Can you work these out from the model? Positions are in its coordinate system, mm. Face numbers are marked on the shaded views. A direction names the side the tool comes from. Coordinates: 2 decimals unless noted, no trailing zeros. Order: outer loops, then holes, each group sorted by start corner. A loop starts at its lowest first (then second) coordinate and runs counter-clockwise, first axis right, second up. Notation, with made-up numbers: (47, 44) -> (96, 44) arc R29 cw to (96, 80) -> close; hole circle Ø3 at (72, 48). An arc over 180 degrees is marked (long way). Use a Markdown table: item, result. Add a question column.
1. Suppose I cut it at C-C, the plane y = 9. State how many separate pieces and enclosed holes the cut face has, then the cut area to 3 significant figures.
2. Suppose I cut it at A-A, the plane z = 11. List the corners of the cut face in (x, y) for me, then the cut area to 3 significant figures.
3. For the marked faces 3, 4 and 5, which set-ups out of +Z, -Z, +X, -X, +Y, -Y let a thin tool reach every point of the face, with its end or its side?
4. Suppose I cut it at D-D, the plane z = -26.5. List the corners of the cut face in (x, y) for me.
5. If I drill on line 1 along Z through (x, y) = (87, 9.75); line 2 along Y through (x, z) = (11, -15.5); line 3 along Y through (x, z) = (52, -1), over which ranges is the centre line in solid material (lowest first)? Write a range as from..to.
6. We'd pull the mould along X, two halves only. Please class the marked faces 1 and 2: pulls with the +X half, pulls with the -X half, needs draft (parallel to the pull), parting line crosses it, or undercut.
7. Suppose I cut it at B-B, the plane x = 64.5. List the corners of the cut face in (y, z) for me.
8. For pin 1 Ø5 at (x, z) = (52, 6.5) entering from +Y; pin 2 Ø0.9 at (x, y) = (67.5, 7) entering from -Z; pin 3 Ø2 at (x, y) = (55, 3) entering from -Z; pin 4 Ø3 at (x, y) = (47.5, 2) entering from +Z, each with a flat end and sliding along its axis, tell me the tip position at first contact or that it passes through.
```python
from build123d import *

# Parameters (mm, degrees)
SKETCH1_W            = 100
SKETCH1_H            = 16
BOSS_EXTRUDE1_DEPTH  = 3
SKETCH2_W            = 98
SKETCH2_H            = 14
CUT_EXTRUDE1_DEPTH   = 1
SKETCH5_W            = 20
SKETCH5_H            = 3
BOSS_EXTRUDE4_DEPTH  = 15
SKETCH6_W            = 20
SKETCH6_H            = 3
BOSS_EXTRUDE5_DEPTH  = 15
FILLET18_R           = 10
SKETCH7_W            = 3
SKETCH7_H            = 12
BOSS_EXTRUDE6_DEPTH  = 17
SKETCH8_W            = 6
SKETCH8_H            = 2
BOSS_EXTRUDE7_DEPTH  = 2
FILLET19_R           = 6
SKETCH10_W           = 60
SKETCH10_H           = 3
BOSS_EXTRUDE8_DEPTH  = 3
SKETCH11_W           = 60
SKETCH11_H           = 3
BOSS_EXTRUDE9_DEPTH  = 3
SKETCH12_W           = 0.95
SKETCH12_H           = 14
BOSS_EXTRUDE10_DEPTH = 3
SKETCH13_W           = 100
SKETCH13_H           = 0.95
BOSS_EXTRUDE11_DEPTH = 3
SKETCH14_W           = 0.95
SKETCH14_H           = 0.052088128
BOSS_EXTRUDE12_DEPTH = 3
SKETCH15_W           = 0.95
SKETCH15_H           = 0.047911872
SKETCH15_W_2         = 0.949734752
SKETCH15_H_2         = 0.052088128
BOSS_EXTRUDE13_DEPTH = 3
FILLET20_R           = 10
SKETCH17_W           = 98.1
SKETCH17_H           = 14.1
SKETCH17_W_2         = 97.1
SKETCH17_H_2         = 13.1
CUT_EXTRUDE2_DEPTH   = 4
SKETCH18_W           = 100
SKETCH18_H           = 16.05
SKETCH18_W_2         = 98
SKETCH18_H_2         = 14.05
CUT_EXTRUDE3_DEPTH   = 2
SKETCH19_W           = 100
SKETCH19_H           = 16
SKETCH19_W_2         = 98.1
SKETCH19_H_2         = 14.1
BOSS_EXTRUDE14_DEPTH = 1


with BuildPart() as part:
    # Sketch1 → Boss-Extrude1 (new body)
    with BuildSketch(Plane(origin=(0, 0, 0), x_dir=(1, 0, 0), z_dir=(0, 1, 0))):
        with Locations((50, 8)):
            Rectangle(SKETCH1_W, SKETCH1_H)
    extrude(amount=BOSS_EXTRUDE1_DEPTH)

    # Sketch2 → Cut-Extrude1 (cut)
    with BuildSketch(Plane(origin=(0, 3, 0), x_dir=(1, 0, 0), z_dir=(0, 1, 0))):
        with Locations((50, 8)):
            Rectangle(SKETCH2_W, SKETCH2_H)
    extrude(amount=-CUT_EXTRUDE1_DEPTH, mode=Mode.SUBTRACT)

    # Sketch5 → Boss-Extrude4 (add)
    with BuildSketch(Plane.XY):
        with Locations((10, 1.5)):
            Rectangle(SKETCH5_W, SKETCH5_H)
        with Locations((90, 1.5)):
            Rectangle(SKETCH5_W, SKETCH5_H)
    extrude(amount=BOSS_EXTRUDE4_DEPTH)

    # Sketch6 → Boss-Extrude5 (add)
    with BuildSketch(Plane(origin=(0, 0, -16), x_dir=(-1, 0, 0), z_dir=(0, 0, -1))):
        with Locations((-90, 1.5)):
            Rectangle(SKETCH6_W, SKETCH6_H)
        with Locations((-10, 1.5)):
            Rectangle(SKETCH6_W, SKETCH6_H)
    extrude(amount=BOSS_EXTRUDE5_DEPTH)

    # Fillet18
    fillet18_edges = [part.edges().sort_by_distance(p)[0] for p in [
        (20, 1.5, 15),
        (0, 1.5, 15),
        (80, 1.5, 15),
        (100, 1.5, 15),
        (0, 1.5, -31),
        (20, 1.5, -31),
        (80, 1.5, -31),
        (100, 1.5, -31),
    ]]
    fillet(fillet18_edges, radius=FILLET18_R - 0.0001)  # a hair under: the kernel refuses the full size

    # Sketch7 → Boss-Extrude6 (add)
    with BuildSketch(Plane(origin=(0, 2, 0), x_dir=(1, 0, 0), z_dir=(0, 1, 0))):
        with Locations((95, 8)):
            Rectangle(SKETCH7_W, SKETCH7_H)
        with Locations((86, 8)):
            Rectangle(SKETCH7_W, SKETCH7_H)
        with Locations((77, 8)):
            Rectangle(SKETCH7_W, SKETCH7_H)
        with Locations((68, 8)):
            Rectangle(SKETCH7_W, SKETCH7_H)
        with Locations((59, 8)):
            Rectangle(SKETCH7_W, SKETCH7_H)
        with Locations((50, 8)):
            Rectangle(SKETCH7_W, SKETCH7_H)
        with Locations((41, 8)):
            Rectangle(SKETCH7_W, SKETCH7_H)
        with Locations((32, 8)):
            Rectangle(SKETCH7_W, SKETCH7_H)
        with Locations((23, 8)):
            Rectangle(SKETCH7_W, SKETCH7_H)
        with Locations((14, 8)):
            Rectangle(SKETCH7_W, SKETCH7_H)
        with Locations((5, 8)):
            Rectangle(SKETCH7_W, SKETCH7_H)
    extrude(amount=BOSS_EXTRUDE6_DEPTH)

    # Sketch8 → Boss-Extrude7 (add)
    with BuildSketch(Plane(origin=(0, 2, 0), x_dir=(1, 0, 0), z_dir=(0, 1, 0))):
        with Locations((90.5, 8)):
            Rectangle(SKETCH8_W, SKETCH8_H)
        with Locations((81.5, 8)):
            Rectangle(SKETCH8_W, SKETCH8_H)
        with Locations((72.5, 8)):
            Rectangle(SKETCH8_W, SKETCH8_H)
        with Locations((63.5, 8)):
            Rectangle(SKETCH8_W, SKETCH8_H)
        with Locations((54.5, 8)):
            Rectangle(SKETCH8_W, SKETCH8_H)
        with Locations((45.5, 8)):
            Rectangle(SKETCH8_W, SKETCH8_H)
        with Locations((36.5, 8)):
            Rectangle(SKETCH8_W, SKETCH8_H)
        with Locations((27.5, 8)):
            Rectangle(SKETCH8_W, SKETCH8_H)
        with Locations((18.5, 8)):
            Rectangle(SKETCH8_W, SKETCH8_H)
        with Locations((9.5, 8)):
            Rectangle(SKETCH8_W, SKETCH8_H)
    extrude(amount=BOSS_EXTRUDE7_DEPTH)

    # Fillet19
    fillet19_edges = [part.edges().sort_by_distance(p)[0] for p in [
        (95, 19, -2),
        (95, 19, -14),
        (86, 19, -2),
        (86, 19, -14),
        (77, 19, -2),
        (77, 19, -14),
        (68, 19, -2),
        (68, 19, -14),
        (59, 19, -2),
        (59, 19, -14),
        (50, 19, -2),
        (50, 19, -14),
        (41, 19, -2),
        (41, 19, -14),
        (32, 19, -2),
        (32, 19, -14),
        (23, 19, -14),
        (23, 19, -2),
        (14, 19, -2),
        (14, 19, -14),
        (5, 19, -2),
        (5, 19, -14),
    ]]
    fillet(fillet19_edges, radius=FILLET19_R - 0.0001)  # a hair under: the kernel refuses the full size

    # Sketch10 → Boss-Extrude8 (add)
    with BuildSketch(Plane(origin=(0, 0, -16), x_dir=(-1, 0, 0), z_dir=(0, 0, -1))):
        with Locations((-50, 1.5)):
            Rectangle(SKETCH10_W, SKETCH10_H)
    extrude(amount=BOSS_EXTRUDE8_DEPTH)

    # Sketch11 → Boss-Extrude9 (add)
    with BuildSketch(Plane.XY):
        with Locations((50, 1.5)):
            Rectangle(SKETCH11_W, SKETCH11_H)
    extrude(amount=BOSS_EXTRUDE9_DEPTH)

    # Sketch12 → Boss-Extrude10 (add)
    with BuildSketch(Plane(origin=(0, 3, 0), x_dir=(1, 0, 0), z_dir=(0, 1, 0))):
        with Locations((99.525, 7.997911872)):
            Rectangle(SKETCH12_W, SKETCH12_H)
        with Locations((0.475, 7.997911872)):
            Rectangle(SKETCH12_W, SKETCH12_H)
    extrude(amount=BOSS_EXTRUDE10_DEPTH)

    # Sketch13 → Boss-Extrude11 (add)
    with BuildSketch(Plane(origin=(0, 3, 0), x_dir=(1, 0, 0), z_dir=(0, 1, 0))):
        with Locations((50, 15.525)):
            Rectangle(SKETCH13_W, SKETCH13_H)
        with Locations((50, 0.475)):
            Rectangle(SKETCH13_W, SKETCH13_H)
    extrude(amount=BOSS_EXTRUDE11_DEPTH)

    # Sketch14 → Boss-Extrude12 (add)
    with BuildSketch(Plane(origin=(0, 3, 0), x_dir=(1, 0, 0), z_dir=(0, 1, 0))):
        with Locations((0.475, 15.023955936)):
            Rectangle(SKETCH14_W, SKETCH14_H)
    extrude(amount=BOSS_EXTRUDE12_DEPTH)

    # Sketch15 → Boss-Extrude13 (add)
    with BuildSketch(Plane(origin=(0, 3, 0), x_dir=(1, 0, 0), z_dir=(0, 1, 0))):
        with Locations((0.475, 0.973955936)):
            Rectangle(SKETCH15_W, SKETCH15_H)
        with Locations((99.525132624, 0.973955936)):
            Rectangle(SKETCH15_W_2, SKETCH15_H)
        with Locations((99.525, 15.023955936)):
            Rectangle(SKETCH15_W, SKETCH15_H_2)
    extrude(amount=BOSS_EXTRUDE13_DEPTH)

    # Fillet20
    fillet20_edges = [part.edges().sort_by_distance(p)[0] for p in [
        (20, 1.5, -19),
        (80, 1.5, -19),
        (80, 1.5, 3),
        (20, 1.5, 3),
    ]]
    fillet(fillet20_edges, radius=FILLET20_R)

    # Sketch17 → Cut-Extrude2 (cut)
    with BuildSketch(Plane(origin=(0, 6, 0), x_dir=(1, 0, 0), z_dir=(0, 1, 0))):
        with Locations((50, 8)):
            Rectangle(SKETCH17_W, SKETCH17_H)
        with Locations((50, 8)):
            Rectangle(SKETCH17_W_2, SKETCH17_H_2, mode=Mode.SUBTRACT)
    extrude(amount=-CUT_EXTRUDE2_DEPTH, mode=Mode.SUBTRACT)

    # Sketch18 → Cut-Extrude3 (cut)
    with BuildSketch(Plane(origin=(0, 6, 0), x_dir=(1, 0, 0), z_dir=(0, 1, 0))):
        with Locations((50, 7.975)):
            Rectangle(SKETCH18_W, SKETCH18_H)
        with Locations((50, 7.975)):
            Rectangle(SKETCH18_W_2, SKETCH18_H_2, mode=Mode.SUBTRACT)
    extrude(amount=-CUT_EXTRUDE3_DEPTH, mode=Mode.SUBTRACT)

    # Sketch19 → Boss-Extrude14 (add)
    with BuildSketch(Plane(origin=(0, 4, 0), x_dir=(1, 0, 0), z_dir=(0, 1, 0))):
        with Locations((50, 8)):
            Rectangle(SKETCH19_W, SKETCH19_H)
        with Locations((50, 8)):
            Rectangle(SKETCH19_W_2, SKETCH19_H_2, mode=Mode.SUBTRACT)
    extrude(amount=BOSS_EXTRUDE14_DEPTH)


solid = part.part
```
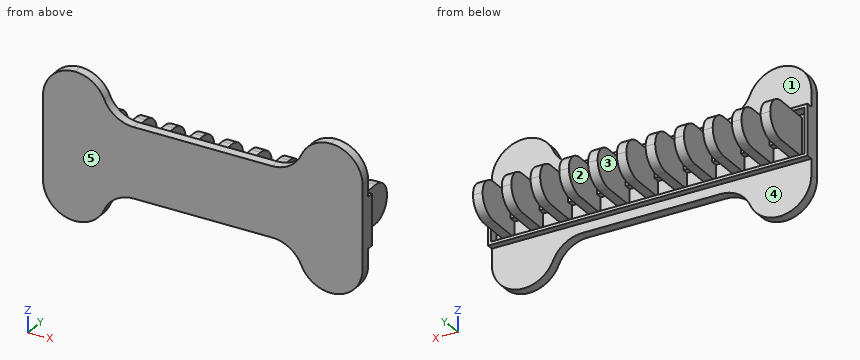
Worked out:
| question | item | result |
|---|---|---|
| 1 | separate pieces | 11 |
| 1 | enclosed holes | 0 |
| 1 | area | 396 mm² |
| 2 | outline | (2, 0) -> (18, 0) -> (18, 3) -> (2, 3) -> close; (82, 0) -> (98, 0) -> (98, 3) -> (82, 3) -> close |
| 2 | area | 96.0 mm² |
| 3 | face 3 | +Y |
| 3 | face 4 | -Z, +X, -X, +Y |
| 3 | face 5 | +Z, -Z, +X, -X, -Y |
| 4 | outline | (1.65, 0) -> (18.35, 0) -> (18.35, 3) -> (1.65, 3) -> close; (81.65, 0) -> (98.35, 0) -> (98.35, 3) -> (81.65, 3) -> close |
| 5 | line 1 | z = -14..-2 |
| 5 | line 2 | y = 0..5 |
| 5 | line 3 | y = 0..2 |
| 6 | face 1 | needs draft |
| 6 | face 2 | undercut |
| 7 | outline | (0, -19) -> (3, -19) -> (3, -16) -> (5, -16) -> (5, -15.05) -> (2, -15.05) -> (2, -9) -> (4, -9) -> (4, -7) -> (2, -7) -> (2, -0.95) -> (5, -0.95) -> (5, 0) -> (3, 0) -> (3, 3) -> (0, 3) -> close |
| 8 | pin 1 | passes through |
| 8 | pin 2 | stops at z = -14 |
| 8 | pin 3 | stops at z = -19 |
| 8 | pin 4 | stops at z = 3 |
